Check sheet for the drawn part. Datum: minimum x, y, z corner. Units: mm. A direction names the side the tool comes from. Coordinates: 2 decimals unless noted, no trailing zeros. Order: outer loops, then holes, each group sorted by start corner. A loop starts at its lowest first (then second) coordinate and runs counter-clockwise, first axis right, second up. Notation, with made-up numbers: (-26.75, 58) -> (27.25, 58) arc R20 cw to (27.25, 72) -> close; hole circle Ø1 at (80, 3). An arc over 180 degrees is marked (long way). Answer as CSV lines item,"result".
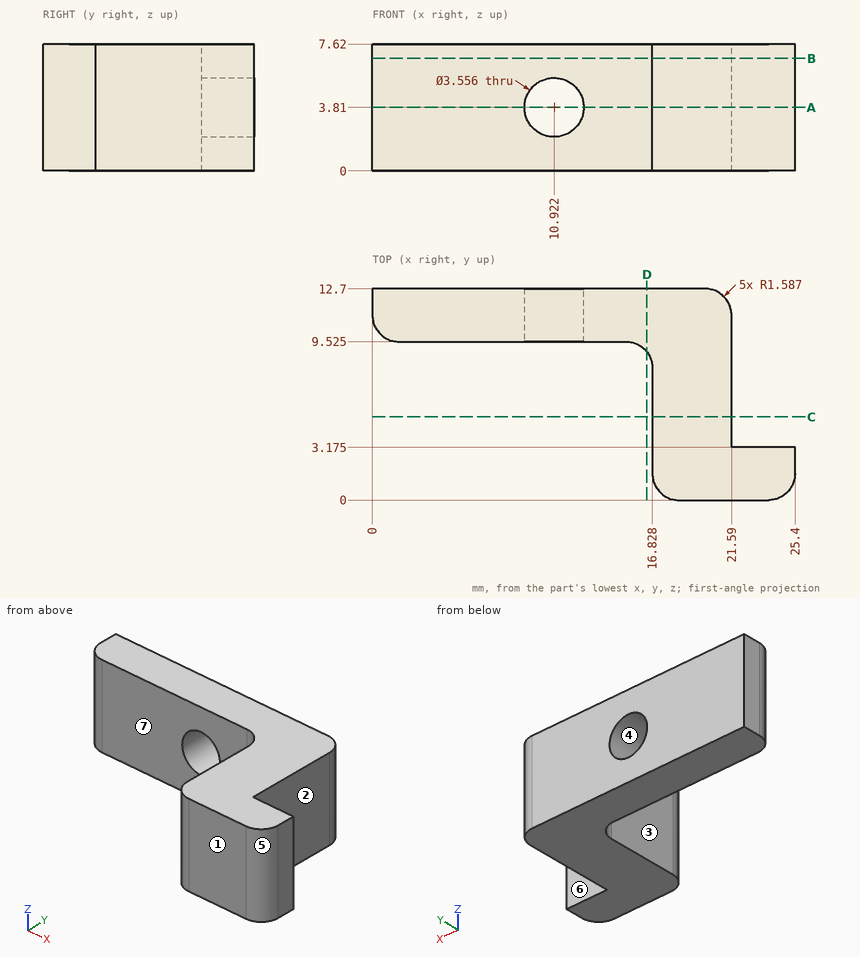
Item 1: Section check B-B, the plane z = 6.75. Record the boundary of the cut face in (x, y) (1 decimal), plus the area to 3 significant figures.
Answer list:
outline,"(0, 11.1) arc R1.6 ccw to (1.6, 9.5) -> (15.2, 9.5) arc R1.6 cw to (16.8, 7.9) -> (16.8, 1.6) arc R1.6 ccw to (18.4, 0) -> (23.8, 0) arc R1.6 ccw to (25.4, 1.6) -> (25.4, 3.2) -> (21.6, 3.2) -> (21.6, 11.1) arc R1.6 ccw to (20, 12.7) -> (0, 12.7) -> close"
area,"124 mm2"
Item 2: Section check C-C, the plane y = 5. Record the boundary of the cut face in (x, z), plus the area to 3 significant figures.
Answer list:
outline,"(16.83, 0) -> (21.59, 0) -> (21.59, 7.62) -> (16.83, 7.62) -> close"
area,"36.3 mm2"
Item 3: Release check for a two-part mould opening along X. For the marked faces 1, 2, 3 and 4 record: +X half, -X half, draft (parallel to the pull), parting line (faces both ways), or undercut.
Answer list:
face 1,"draft"
face 2,"+X half"
face 3,"-X half"
face 4,"undercut"
Item 4: Tool access check on the marked faces 5, 6 and 7. Record the directions out of +Z, -Z, +X, -X, +Y, -Y that give a thin tool (end or side, any length) a straight path to the whole face; none if there is none.
Answer list:
face 5,"+Z, -Z, +X, -Y"
face 6,"+Z, -Z, +X, +Y"
face 7,"+Z, -Z, -X, -Y"
Item 5: Section check D-D, the plane x = 16.5. Record the boundary of the cut face in (y, z).
Answer list:
outline,"(8.9, 0) -> (12.7, 0) -> (12.7, 7.62) -> (8.9, 7.62) -> close"
Item 6: Thickness scan on line 1 (Y direction, x = 21.75, z = 1.75) (1 decimal); line 2 (X direction, y = 8, z = 1); line 3 (Y direction, x = 13, z = 5.5) (1 decimal). Record the ranges inside material, lowest first.
Answer list:
line 1,"0 to 3.2"
line 2,"16.83 to 21.59"
line 3,"9.5 to 12.7"
Item 7: Section check A-A, the plane z = 3.81. Record the boundary of the cut face in (x, y) (1 decimal).
Answer list:
outline,"(0, 11.1) arc R1.6 ccw to (1.6, 9.5) -> (9.1, 9.5) -> (9.1, 12.7) -> (0, 12.7) -> close; (12.7, 9.5) -> (15.2, 9.5) arc R1.6 cw to (16.8, 7.9) -> (16.8, 1.6) arc R1.6 ccw to (18.4, 0) -> (23.8, 0) arc R1.6 ccw to (25.4, 1.6) -> (25.4, 3.2) -> (21.6, 3.2) -> (21.6, 11.1) arc R1.6 ccw to (20, 12.7) -> (12.7, 12.7) -> close"
Item 8: Depth check by flat-ended pin: pin 1 Ø4 at (y, z) = (10, 6) entering from +X; pin 2 Ø1.9 at (y, z) = (3, 3) entering from -X; pin 3 Ø1.1 at (x, z) = (23, 5.5) entering from +Y (1 decimal); pin 4 Ø4.5 at (x, z) = (10.922, 3.81) entering from +Y. Enter the tip coordinate at first touch or a pass-through.
Answer list:
pin 1,"x = 21.59"
pin 2,"x = 16.83"
pin 3,"y = 3.2"
pin 4,"y = 12.7"
